from build123d import *

# Parameters (mm, degrees)
BOSS_EXTRUDE1_DEPTH             = 160
RIB3_REACH                      = 111.505
SKETCH4_WALL_W                  = 239.367706636
SKETCH4_WALL_H                  = 3
RIB4_START                      = -3
RIB4_DEPTH                      = 3
F_6_CLEARANCE_HOLE1_D           = 3.7973
TAP_DRILL_FOR_M3X0_5_TAP1_D     = 2.5
TAP_DRILL_FOR_M3X0_5_TAP1_DEPTH = 5
TAP_DRILL_FOR_M3X0_5_TAP1_TIP   = 0.751075774


# Read off the part's stored shape, not the designer's step: Rib4
with BuildPart() as part:
    # Sketch1 → Boss-Extrude1 (new body)
    with BuildSketch(Plane.XY):
        with BuildLine():
            Line((0, 0), (0, 12))
            Line((0, 12), (-8, 12))
            Line((-8, 12), (-8, 6))
            ThreePointArc((-8, 6), (-8.878679656, 3.878679656), (-11, 3))
            Line((-11, 3), (-24, 3))
            Line((-24, 3), (-24, 0))
            Line((-24, 0), (0, 0))
        make_face()
    extrude(amount=BOSS_EXTRUDE1_DEPTH)

    # Sketch4 wall → Rib3 (add, up to next)
    with BuildSketch(Plane(origin=(-16, 7.5, 53.83333334), x_dir=(-0.871575537125, -0.490261239633, 0), z_dir=(-0.490261239633, 0.871575537125, 0)), mode=Mode.PRIVATE) as rib3_sk1:
        Rectangle(SKETCH4_WALL_W, SKETCH4_WALL_H)
    rib3_tool1 = extrude(rib3_sk1.sketch, amount=-RIB3_REACH, mode=Mode.PRIVATE) - part.part
    rib3 = rib3_tool1.solids().sort_by_distance((-16, 7.5, 53.83333334))[0]
    add(rib3)

    # Rib4 outline → Rib4 (add)
    with BuildSketch(Plane(origin=(0, 0, 0), x_dir=(-1, 0, 0), z_dir=(0, 0, -1)).offset(RIB4_START)):
        with BuildLine():
            Line((24, 3), (8, 12))
            Line((8, 12), (8, 6))
            ThreePointArc((8, 6), (8.878679656, 3.878679656), (11, 3))
            Line((11, 3), (24, 3))
        make_face()
    rib4 = extrude(amount=RIB4_DEPTH)

    # Mirror1: Rib3, Rib4 across plane
    add(rib3.mirror(Plane(origin=(0, 0, 80), x_dir=(1, 0, 0), z_dir=(0, 0, -1))))
    add(rib4.mirror(Plane(origin=(0, 0, 80), x_dir=(1, 0, 0), z_dir=(0, 0, -1))))

    # 6 Clearance Hole1 (through all)
    with Locations(Plane(origin=(0, 0, 0), x_dir=(-1, 0, 0), z_dir=(0, -1, 0))):
        with Locations((17.49975, -10), (17.49975, -80), (17.49975, -150)):
            Hole(F_6_CLEARANCE_HOLE1_D / 2)

    # Tap Drill for M3x0.5 Tap1
    with Locations(Plane(origin=(0, 0, 0), x_dir=(-1, 0, 0), z_dir=(0, -1, 0))):
        with Locations((4.249875, -42.33333334), (4.249875, -117.66666666)):
            Hole(TAP_DRILL_FOR_M3X0_5_TAP1_D / 2, depth=TAP_DRILL_FOR_M3X0_5_TAP1_DEPTH)
            with Locations((0, 0, -(TAP_DRILL_FOR_M3X0_5_TAP1_DEPTH + TAP_DRILL_FOR_M3X0_5_TAP1_TIP / 2))):  # 118° drill point
                Cone(0, TAP_DRILL_FOR_M3X0_5_TAP1_D / 2, TAP_DRILL_FOR_M3X0_5_TAP1_TIP, mode=Mode.SUBTRACT)


solid = part.part
Part model, mm, in its own coordinate system. A direction names the side the tool comes from. Coordinates: 2 decimals unless noted, no trailing zeros. Order: outer loops, then holes, each group sorted by start corner. A loop starts at its lowest first (then second) coordinate and runs counter-clockwise, first axis right, second up.
(1) Probe L1, parallel to Z at x = -11.25, y = 8.5; L2, parallel to Z at x = -16.75, y = 1.75; L3, parallel to X at y = 1.65, z = 80. List the from-to ranges inside material, lowest first.
Check sheet entries:
L1: z = 0 to 3, 52.33 to 55.33, 104.67 to 107.67, 157 to 160
L2: z = 0 to 8.26, 11.74 to 78.26, 81.74 to 148.26, 151.74 to 160
L3: x = -24 to -19.4, -15.6 to 0
(2) Slice it at C-C, the plane x = -12.5. Write the cut outline in (y, z), and give its area (3 significant figures).
Check sheet entries:
outline: (0, 0) - (9.47, 0) - (9.47, 3) - (3, 3) - (3, 52.33) - (9.47, 52.33) - (9.47, 55.33) - (3, 55.33) - (3, 104.67) - (9.47, 104.67) - (9.47, 107.67) - (3, 107.67) - (3, 157) - (9.47, 157) - (9.47, 160) - (0, 160) - close
area: 558 mm2
(3) Slice it at B-B, the plane z = 22.5. Write the cut outline in (x, y).
Check sheet entries:
outline: (-24, 0) - (0, 0) - (0, 12) - (-8, 12) - (-8, 6) arc R3 cw to (-11, 3) - (-24, 3) - close
(4) Tool access for faces 4 (the face through (-3.6, 2.5, 116.6)), 5 (the face through (-15.89, 7.56, 53.85)), 6 (the face through (-8, 9, 80)): list every direction of +Z, -Z, +X, -X, +Y, -Y with a clear straight run to the whole face (end or side of a thin tool).
Check sheet entries:
face 4: -Y
face 5: +Z, -Z, -X, +Y
face 6: -X, +Y
(5) Pin check, flat tips, straight feed: pin 1 Ø10.5 at (x, z) = (-14.5, 122.5) entering from +Y; pin 2 Ø5 at (x, z) = (-17.5, 80) entering from +Y; pin 3 Ø6.5 at (y, z) = (8.5, 30) entering from -X. Stop position of each tip, or through.
Check sheet entries:
pin 1: stops at y = 3.56
pin 2: stops at y = 3
pin 3: stops at x = -8.1
(6) Slice it at A-A, the plane z = 80. Write the cut outline in (x, y), and give its area (3 significant figures).
Check sheet entries:
outline: (-24, 0) - (-19.4, 0) - (-19.4, 3) - (-24, 3) - close; (-15.6, 0) - (0, 0) - (0, 12) - (-8, 12) - (-8, 6) arc R3 cw to (-11, 3) - (-15.6, 3) - close
area: 135 mm2
(7) Pull direction Z, two halves, no side cores. Call faces 1 (the face through (-16.11, 7.44, 1.52)), 2 (the face through (-8.86, 3.9, 27.32)), 3 (the face through (-9, 5, 160)): pulls with the +Z half, pulls with the -Z half, needs draft (parallel to the pull), parting line crosses it, or undercut.
Check sheet entries:
face 1: needs draft
face 2: undercut
face 3: pulls with the +Z half
